from build123d import *

# Parameters (mm, degrees)
SKETCH1_R           = 7.5
BOSS_EXTRUDE1_DEPTH = 5
SKETCH2_R           = 1.75
BOSS_EXTRUDE2_DEPTH = 5
CIRPATTERN3_COUNT   = 2
FILLET5_R           = 0.5


with BuildPart() as part:
    # Sketch1 → Boss-Extrude1 (new body)
    with BuildSketch(Plane(origin=(0, 0, 0), x_dir=(1, 0, 0), z_dir=(0, 1, 0))):
        with Locations(Location((0, 0, 0), (0, 0, 270))):
            Circle(SKETCH1_R)
    extrude(amount=BOSS_EXTRUDE1_DEPTH)

    # Sketch2 → Boss-Extrude2 (add)
    with BuildSketch(Plane(origin=(0, 0, 0), x_dir=(1, 0, 0), z_dir=(0, 1, 0))):
        with BuildLine():
            Line((12.716294884, 4.995006753), (21.973895335, 12.630243088))
            ThreePointArc((21.973895335, 12.630243088), (22.551056235, 19.785091931), (15.381932825, 20.143764773))
            Line((15.381932825, 20.143764773), (6.607081232, 11.958291083))
            ThreePointArc((6.607081232, 11.958291083), (4.300797699, 10.454751027), (1.621374113, 9.822085487))
            ThreePointArc((1.621374113, 9.822085487), (-2.205943818, 8.582985268), (-4.946272983, 5.637764059))
            Line((-4.946272983, 5.637764059), (0, 0))
            Line((0, 0), (4.946272983, -5.637764059))
            ThreePointArc((4.946272983, -5.637764059), (8.223006092, -3.303936295), (9.949550947, 0.329625974))
            ThreePointArc((9.949550947, 0.329625974), (10.925462035, 2.903955787), (12.716294884, 4.995006753))
        make_face()
        with Locations(Location((18.792546862, 16.487576609, 0), (0, 0, 270))):
            Circle(SKETCH2_R, mode=Mode.SUBTRACT)
    boss_extrude2 = extrude(amount=-BOSS_EXTRUDE2_DEPTH)

    # CirPattern3: Boss-Extrude2 ×2 about axis
    cirpattern3_axis = Axis((0, 0, 0), (0, 1, 0))
    for i in range(1, CIRPATTERN3_COUNT):
        add(boss_extrude2.rotate(cirpattern3_axis, i * 360 / CIRPATTERN3_COUNT))

    # Fillet5
    fillet5_edges = [part.edges().sort_by_distance(p)[0] for p in [
        (0, 5, -7.5),
    ]]
    fillet(fillet5_edges, radius=FILLET5_R)


solid = part.part
Source: CAD feature listing. Evaluate the final solid. Frame: model axes, mm. A direction names the side the tool comes from. Give positions to 0.01 mm unless a question says otherwise; leave off trailing zeros. Write each loop counter-clockwise with the first axis right and the second up, starting at its lowest first coordinate (ties: lowest second). Pieces come first, ordered by that corner, then holes. Notation, with made-up numbers: (6.25, 84.5) -> (65.25, 84.5) arc R19 cw to (65.25, 115.5) -> close; hole circle Ø11 at (-15.5, 36.5). An arc over 180 degrees is marked (long way). Write item = value, one per line.
Q1. First-contact query: pin 1 (6 mm diameter, centred on x = -7, y = -2, fed in from +Z); pin 2 (6 mm diameter, centred on y = -1, z = -5, fed in from -X); pin 3 (4 mm diameter, centred on y = 1, z = 15, fed in from +X). Flat tips, straight axial feed; report the tip coordinate or a pass-through.
Here are the results:
pin_1 = 15.12
pin_2 = -9.11
pin_3 = -8.01
Q2. Mould query, pull axis Z, two halves, no side actions, for faces 1 (the face through (17.084, -2.465, -16.867)), 2 (the face through (17.28, -2.46, -8.76)), 3 (the face through (-13, 0, 11)). Classes: +Z half, -Z half, draft (parallel to the pull), parting line (faces both ways), or undercut.
Here are the results:
face_1 = undercut
face_2 = +Z half
face_3 = draft
Q3. Cut plane A-A on y = -3.75. Return loops of the section in (x, z) (3 decimals), then the cut area to 3 significant figures.
Here are the results:
outline = (-21.974, 12.63) -> (-12.716, 4.995) arc R8 cw to (-9.95, 0.33) arc R8 ccw to (-4.946, -5.638) arc R8 ccw to (1.621, -9.822) arc R8 cw to (6.607, -11.958) -> (15.382, -20.144) arc R5 ccw (long way) to (21.974, -12.63) -> (12.716, -4.995) arc R8 cw to (9.95, -0.33) arc R8 ccw to (4.946, 5.638) arc R8 ccw to (-1.621, 9.822) arc R8 cw to (-6.607, 11.958) -> (-15.382, 20.144) arc R5 ccw (long way) to start; hole circle Ø3.5 at (-18.793, 16.488); hole circle Ø3.5 at (18.793, -16.488)
area = 633 mm²
Q4. Cut plane D-D on x = 11.5. Return loops of the section in (y, z).
Here are the results:
outline = (-5, -16.52) -> (0, -16.52) -> (0, -3.75) -> (-5, -3.75) -> close
Q5. Line query: line 1 (Y direction, x = -17, z = 17); line 2 (X direction, y = -0.5, z = 8); line 3 (Z direction, x = 17.5, y = -4.5). Output: solid intervals per line, ascending. Write a range as from..to.
Here are the results:
line_1 = -5..0
line_2 = -16.36..3.01
line_3 = -21.32..-17.67, -15.31..-8.94
Q6. Cut plane B-B on x = 0. Return loops of the section in (y, z), then the cut area to 3 significant figures.
Here are the results:
outline = (-5, -9.56) -> (0, -9.56) -> (0, -7.5) -> (4.5, -7.5) arc R0.5 ccw to (5, -7) -> (5, 7) arc R0.5 ccw to (4.5, 7.5) -> (0, 7.5) -> (0, 9.56) -> (-5, 9.56) -> close
area = 170 mm²
Q7. Cut plane C-C on y = 1.75. Return loops of the section in (x, z), then the cut area to 3 significant figures.
Here are the results:
outline = circle Ø15 at (0, 0)
area = 177 mm²
Q8. Reachability of faces 4 (the face through (0.33, 2.218, -7.493)), 5 (the face through (-22.624, -2.465, 19.7)) from +Z, -Z, +X, -X, +Y, -Y: full face, straight path, thin tool, end or side. Return the list, or none.
Here are the results:
face_4 = +Y
face_5 = +Y, -Y
